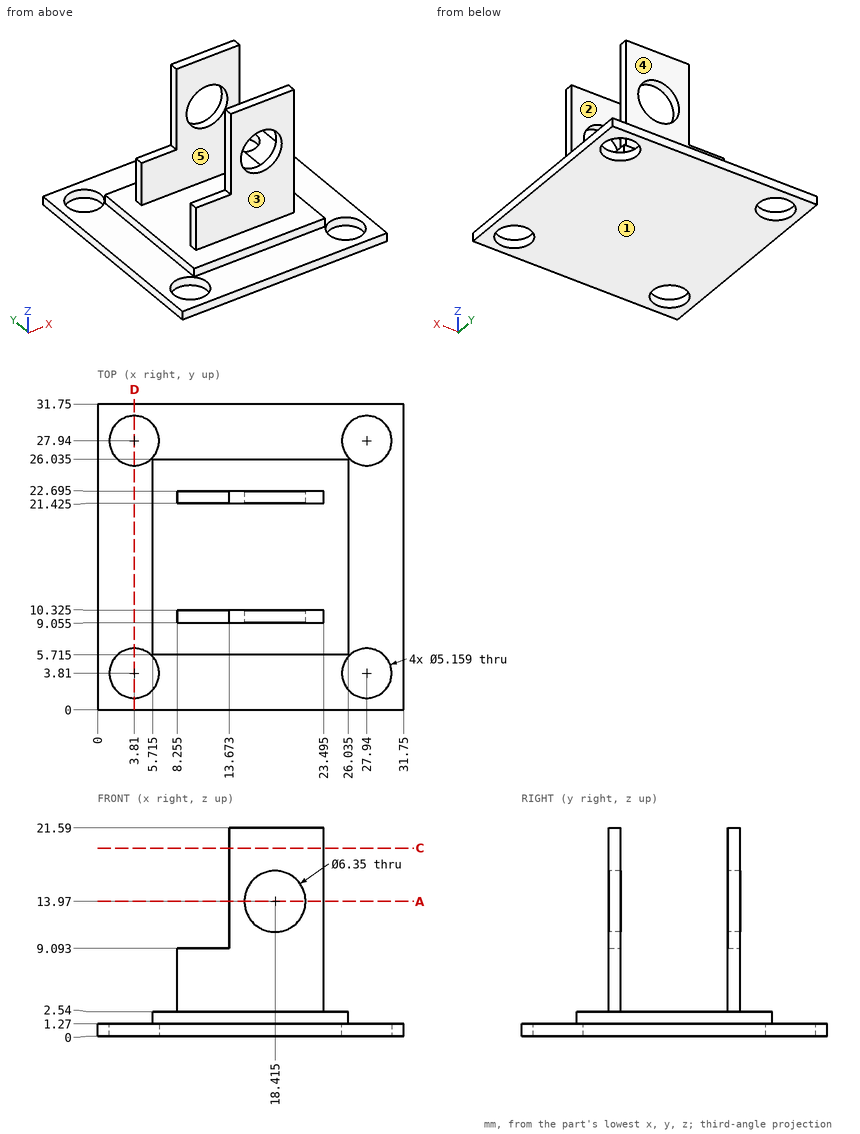
Source: three-view drawing plus pictorial views. Frame: mm from the lowest corner of the part. A direction names the side the tool comes from. Coordinates: 2 decimals unless noted, no trailing zeros. Loops run counter-clockwise (first coordinate to the right, second up) from the corner with the lowest first, then second, coordinate; pieces in that order, holes last. Notation, with made-up numbers: (27, 16.5) - (73, 16.5) arc R24 cw to (73, 38.5) - close; hole circle Ø9 at (71, 80.5). An arc over 180 degrees is marked (long way). Answer in a Markdown table with one row per item. Add a question column.
Item 1: Line query: line 1 along Y through (x, z) = (3.81, 0.3); line 2 along Y through (x, z) = (15.5, 16.25) (1 decimal); line 3 along Z through (x, y) = (14.5, 7.5). Output: solid intervals per line, ascending. Write a range as [from, to].
Item 2: Contact query for flat-ended pins moving along their axis: P1, Ø5, axis at x = 11.5, z = 12, coming from the -Y side (1 decimal); P2, Ø8, axis at x = 28, y = 17, coming from the +Z side; P3, Ø12, axis at x = 9, z = 18, coming from the +Y side (1 decimal). Output: stop coordinate, or through.
Item 3: Section query C-C on z = 19.5. Return the cut outline in (x, y) (1 decimal).
Item 4: Mould query, pull axis Y, two halves, no side actions, for the marked faces 1, 2 and 3. Classes: released by +Y, released by -Y, zero draft, split by the parting line, or undercut.
Item 5: Section query A-A on z = 13.97. Return the cut outline in (x, y) (1 decimal).
Item 6: Access query for the marked faces 4 and 5. Directions: +Z, -Z, +X, -X, +Y, -Y. A direction counts if a zero-diameter tool reaches every point of the face in a straight line with its end or side. Return the directions, or none.
Item 7: Section query D-D on x = 3.81. Return the cut outline in (y, z).
Recorded:
| question | item | result |
|---|---|---|
| 1 | line 1 | [0, 1.23], [6.39, 25.36], [30.52, 31.75] |
| 1 | line 2 | [9.1, 10.3], [21.4, 22.7] |
| 1 | line 3 | [0, 2.54] |
| 2 | P1 | y = 9.1 |
| 2 | P2 | z = 2.54 |
| 2 | P3 | y = 22.7 |
| 3 | outline | (13.7, 9.1) - (23.5, 9.1) - (23.5, 10.3) - (13.7, 10.3) - close; (13.7, 21.4) - (23.5, 21.4) - (23.5, 22.7) - (13.7, 22.7) - close |
| 4 | face 1 | zero draft |
| 4 | face 2 | undercut |
| 4 | face 3 | released by -Y |
| 5 | outline | (13.7, 9.1) - (15.2, 9.1) - (15.2, 10.3) - (13.7, 10.3) - close; (13.7, 21.4) - (15.2, 21.4) - (15.2, 22.7) - (13.7, 22.7) - close; (21.6, 9.1) - (23.5, 9.1) - (23.5, 10.3) - (21.6, 10.3) - close; (21.6, 21.4) - (23.5, 21.4) - (23.5, 22.7) - (21.6, 22.7) - close |
| 6 | face 4 | +Z, +X, -X, +Y |
| 6 | face 5 | +Z, +X, -X |
| 7 | outline | (0, 0) - (1.23, 0) - (1.23, 1.27) - (0, 1.27) - close; (6.39, 0) - (25.36, 0) - (25.36, 1.27) - (6.39, 1.27) - close; (30.52, 0) - (31.75, 0) - (31.75, 1.27) - (30.52, 1.27) - close |
